Check sheet for the modelled part. Datum: model origin and axes. Units: mm. A direction names the side the tool comes from. Give positions to 0.01 mm unless a question says otherwise; leave off trailing zeros. Write each loop counter-clockwise with the first axis right and the second up, starting at its lowest first coordinate (ties: lowest second). Pieces come first, ordered by that corner, then holes. Notation, with made-up numbers: M 19,54.25 L 25,54.25 A13 ccw 25,61.25 Z; hole C -35.75,79 d9. An arc over 180 degrees is marked long. Use CSV: the item, a comma, the result in double quotes. Start each with the question number.
1. Scan lines: line 1 (Y direction, x = -47.5, z = 37.85); line 2 (X direction, y = -5, z = 38.5); line 3 (X direction, y = 27.5, z = 37.95). Record each from-to range of solid material in increasing order.
2. Access from +Z, -Z, +X, -X, +Y, -Y to the whole of each face (thin tool, end or side, straight path). Record for faces 1 (the face through (-52.5, 0, 35)), 2 (the face through (-33, -9.932, 38)), 3 (the face through (-50, -30, 37)).
3. Cross-section at A-A, the plane y = 1.5. Enter the section's corners in (x, z).
4. Cross-section at D-D, the plane z = 33.25. Enter the section's corners in (x, y), and give its area (3 significant figures).
5. Depth check by flat-ended pin: P1, Ø3.5, axis at x = -48.5, y = -28.5, coming from the -Z side; P2, Ø3.5, axis at x = 47.5, y = -27.5, coming from the +Z side. Enter the tip coordinate at first touch or a pass-through.
6. Cross-section at B-B, the plane x = -34. Enter the section's corners in (y, z).
7. Mould release check, pull along Y, two halves, no side actions. Record for faces 4 (the face through (-16, -31, 30)), 5 (the face through (-1, -32.5, 35)), 6 (the face through (0, 0, 38)): +Y half, -Y half, draft (parallel to the pull), parting line (faces both ways), or undercut.
8. Cross-section at C-C, the plane x = 10. Enter the section's corners in (y, z), and give its area (3 significant figures).
from build123d import *

# Parameters (mm, degrees)
SKETCH007_W   = 105
SKETCH007_H   = 10
PAD006_DEPTH  = 2
FILLET006_R   = 1
SKETCH008_W   = 105
SKETCH008_H   = 10
PAD007_DEPTH  = 2
FILLET012_R   = 1
FILLET014_R   = 1
FILLET023_R   = 1
SKETCH009_W   = 65
SKETCH009_H   = 10
PAD008_DEPTH  = 2
FILLET013_R   = 1
FILLET020_R   = 1
FILLET027_R   = 1
SKETCH010_W   = 65
SKETCH010_H   = 10
PAD009_DEPTH  = 2
FILLET007_R   = 1
FILLET011_R   = 1
FILLET025_R   = 1
SKETCH006_W   = 105
SKETCH006_H   = 65
SKETCH006_R   = 3
SKETCH006_R_2 = 1
SKETCH006_W_2 = 15
SKETCH006_H_2 = 20
SKETCH006_W_3 = 20
SKETCH006_H_3 = 15
PAD005_DEPTH  = 3


with BuildPart() as body006:
    # Sketch007 → Pad006 (new body)
    with BuildSketch(Plane.XZ):
        with Locations((0, 5)):
            Rectangle(SKETCH007_W, SKETCH007_H)
    extrude(amount=PAD006_DEPTH)

    # Fillet006
    fillet006_edges = [body006.edges().sort_by_distance(p)[0] for p in [
        (52.5, -2, 5),
    ]]
    fillet(fillet006_edges, radius=FILLET006_R)


with BuildPart() as body006_1:
    # Body006 placement: moved
    add(body006.part.moved(Location((0, -30.5, 36))))


with BuildPart() as body007:
    # Sketch008 → Pad007 (new body)
    with BuildSketch(Plane.XZ):
        with Locations((0, 5)):
            Rectangle(SKETCH008_W, SKETCH008_H)
    extrude(amount=PAD007_DEPTH)

    # Fillet012
    fillet012_edges = [body007.edges().sort_by_distance(p)[0] for p in [
        (52.5, 0, 5),
    ]]
    fillet(fillet012_edges, radius=FILLET012_R)

    # Fillet014
    fillet014_edges = [body007.edges().sort_by_distance(p)[0] for p in [
        (-52.5, 0, 5),
    ]]
    fillet(fillet014_edges, radius=FILLET014_R)

    # Fillet023
    fillet023_edges = [body007.edges().sort_by_distance(p)[0] for p in [
        (0, 0, 10),
    ]]
    fillet(fillet023_edges, radius=FILLET023_R)


with BuildPart() as body007_1:
    # Body007 placement: moved
    add(body007.part.moved(Location((0, 32.5, 36))))


with BuildPart() as body008:
    # Sketch009 → Pad008 (new body)
    with BuildSketch(Plane.YZ):
        with Locations((0, 5)):
            Rectangle(SKETCH009_W, SKETCH009_H)
    extrude(amount=PAD008_DEPTH)

    # Fillet013
    fillet013_edges = [body008.edges().sort_by_distance(p)[0] for p in [
        (0, 32.5, 5),
    ]]
    fillet(fillet013_edges, radius=FILLET013_R)

    # Fillet020
    fillet020_edges = [body008.edges().sort_by_distance(p)[0] for p in [
        (0, -32.5, 5),
    ]]
    fillet(fillet020_edges, radius=FILLET020_R)

    # Fillet027
    fillet027_edges = [body008.edges().sort_by_distance(p)[0] for p in [
        (0, 0, 10),
    ]]
    fillet(fillet027_edges, radius=FILLET027_R)


with BuildPart() as body008_1:
    # Body008 placement: moved
    add(body008.part.moved(Location((-52.5, 0, 36))))


with BuildPart() as body009:
    # Sketch010 → Pad009 (new body)
    with BuildSketch(Plane.YZ):
        with Locations((0, 5)):
            Rectangle(SKETCH010_W, SKETCH010_H)
    extrude(amount=PAD009_DEPTH)

    # Fillet007
    fillet007_edges = [body009.edges().sort_by_distance(p)[0] for p in [
        (2, -32.5, 5),
    ]]
    fillet(fillet007_edges, radius=FILLET007_R)

    # Fillet011
    fillet011_edges = [body009.edges().sort_by_distance(p)[0] for p in [
        (2, 32.5, 5),
    ]]
    fillet(fillet011_edges, radius=FILLET011_R)

    # Fillet025
    fillet025_edges = [body009.edges().sort_by_distance(p)[0] for p in [
        (2, 0, 10),
    ]]
    fillet(fillet025_edges, radius=FILLET025_R)


with BuildPart() as body009_1:
    # Body009 placement: moved
    add(body009.part.moved(Location((50.5, 0, 36))))


with BuildPart() as fusion:
    # Sketch006 → Pad005 (new body)
    with BuildSketch(Plane.XY):
        Rectangle(SKETCH006_W, SKETCH006_H)
        with Locations((-47.5, 27.5)):
            Circle(SKETCH006_R, mode=Mode.SUBTRACT)
        with Locations((47.5, 27.5)):
            Circle(SKETCH006_R, mode=Mode.SUBTRACT)
        with Locations((-47.5, -27.5)):
            Circle(SKETCH006_R, mode=Mode.SUBTRACT)
        with Locations((47.5, -27.5)):
            Circle(SKETCH006_R, mode=Mode.SUBTRACT)
        with Locations((10, -10)):
            Circle(SKETCH006_R_2, mode=Mode.SUBTRACT)
        with Locations((-32.489298, 0.067564)):
            Rectangle(SKETCH006_W_2, SKETCH006_H_2, mode=Mode.SUBTRACT)
        with Locations((10, 0.066365)):
            Rectangle(SKETCH006_W_3, SKETCH006_H_3, mode=Mode.SUBTRACT)
    extrude(amount=PAD005_DEPTH)


with BuildPart() as fusion_1:
    # Body005 placement: moved
    add(fusion.part.moved(Location((0, 0, 43))))

    # Fusion: union Body006, Body007, Body008, Body009
    add(body006_1.part)
    add(body007_1.part)
    add(body008_1.part)
    add(body009_1.part)


with BuildPart() as fusion_2:
    # Fusion placement: moved
    add(fusion_1.part.moved(Location((0, 0, -6))))


solid = fusion_2.part
Worked answers:
1,line 1,"y = -32.5 to -30.5, -24.5 to 24.5, 30.5 to 32.5"
1,line 2,"x = -52.5 to -39.99, -24.99 to 0, 20 to 52.5"
1,line 3,"x = -52.5 to -50.5, -44.5 to 44.5, 50.5 to 52.5"
2,face 1,"+Z, -Z, -X, +Y, -Y"
2,face 2,"+Z, -Z"
2,face 3,"-Z"
3,outline,"M -52.5,30 L -50.5,30 L -50.5,37 L -39.99,37 L -39.99,40 L -52.5,40 Z; M -24.99,37 L 0,37 L 0,40 L -24.99,40 Z; M 20,37 L 50.5,37 L 50.5,30 L 52.5,30 L 52.5,40 L 20,40 Z"
4,outline,"M -52.5,-32.5 L 51.5,-32.5 A1 ccw 52.5,-31.5 L 52.5,31.5 A1 ccw 51.5,32.5 L -51.5,32.5 A1 ccw -52.5,31.5 Z; hole M -50.5,-30.5 L 50.5,-30.5 L 50.5,30.5 L -50.5,30.5 Z"
4,area,"663 mm^2"
5,P1,"stops at z = 37"
5,P2,"passes through"
6,outline,"M -32.5,30 L -30.5,30 L -30.5,37 L -9.93,37 L -9.93,40 L -32.5,40 Z; M 10.07,37 L 30.5,37 L 30.5,30 L 32.5,30 L 32.5,40 L 10.07,40 Z"
7,face 4,"draft"
7,face 5,"-Y half"
7,face 6,"undercut"
8,outline,"M -32.5,30 L -30.5,30 L -30.5,37 L -11,37 L -11,40 L -32.5,40 Z; M -9,37 L -7.43,37 L -7.43,40 L -9,40 Z; M 7.57,37 L 30.5,37 L 30.5,30 L 32.5,30 L 32.5,40 L 7.57,40 Z"
8,area,"172 mm^2"
